Source: CAD feature listing. Evaluate the final solid. Frame: model axes, mm. A direction names the side the tool comes from. Round coordinates to 2 decimals unless told otherwise and drop trailing zeros. Loops run counter-clockwise (first coordinate to the right, second up) from the corner with the lowest first, then second, coordinate; pieces in that order, holes last. Notation, with made-up numbers: M 64.25,-4 L 112.25,-4 A17 ccw 112.25,14 Z; hole C 28,8 d1. An arc over 180 degrees is marked long. Answer as a JSON object with one key per item and string values.
from build123d import *

# Parameters (mm, degrees)
SKETCH2_R           = 63.5
BOSS_EXTRUDE1_DEPTH = 25.4
SHELL1_T            = -2
BOSS_EXTRUDE2_DEPTH = 23.4
CUT_EXTRUDE2_DEPTH  = 23.4


with BuildPart() as part:
    # Sketch2 → Boss-Extrude1 (new body)
    with BuildSketch(Plane(origin=(0, 0, 0), x_dir=(0, 1, 0), z_dir=(0, 0, 1))):
        with Locations(Location((0, 0, 0), (0, 0, 270))):
            Circle(SKETCH2_R)
    extrude(amount=BOSS_EXTRUDE1_DEPTH)

    # Shell1
    shell1_openings = [part.faces().sort_by_distance(p)[0] for p in [
        (0, 0, 25.4),
    ]]
    offset(amount=SHELL1_T, openings=shell1_openings, kind=Kind.INTERSECTION)

    # Sketch3 → Boss-Extrude2 (add)
    with BuildSketch(Plane.XY.offset(2)):
        with BuildLine():
            Line((32.449501385, 1.811038348), (34.452433007, 1.811038348))
            ThreePointArc((34.452433007, 1.811038348), (-34.49308373, 0.690778407), (34.352300121, -3.188961652))
            Line((34.352300121, -3.188961652), (32.343168113, -3.188961652))
            ThreePointArc((32.343168113, -3.188961652), (-32.492653095, 0.691010021), (32.449501385, 1.811038348))
        make_face()
    extrude(amount=BOSS_EXTRUDE2_DEPTH)

    # Sketch4 → Cut-Extrude2 (cut)
    with BuildSketch(Plane.XY.offset(25.4)):
        Polygon((34.352300121, -3.188961652), (63.419874831, -3.188961652), (70.082181446, -0.688961652), (63.474169078, 1.811038348), (34.452433007, 1.811038348), align=None)
    extrude(amount=-CUT_EXTRUDE2_DEPTH, mode=Mode.SUBTRACT)


solid = part.part
Item 1: Section A-A on z = 15.5. Return the cut outline in (x, y), then the cut area to 3 significant figures.
Answer sheet:
{"outline": "M 32.34,-3.19 A32.5 cw long 32.45,1.81 L 34.45,1.81 A34.5 ccw long 34.35,-3.19 Z; M 61.42,-3.19 A61.5 cw long 61.47,1.81 L 63.47,1.81 A63.5 ccw long 63.42,-3.19 Z", "area": "1,190 mm²"}
Item 2: Section C-C on x = 0. Return the cut outline in (y, z).
Answer sheet:
{"outline": "M -63.5,0 L 63.5,0 L 63.5,25.4 L 61.5,25.4 L 61.5,2 L 34.5,2 L 34.5,25.4 L 32.5,25.4 L 32.5,2 L -32.5,2 L -32.5,25.4 L -34.5,25.4 L -34.5,2 L -61.5,2 L -61.5,25.4 L -63.5,25.4 Z"}
Item 3: Pull-direction query (X, two-part tool) for faces 1 (the flat face through (-52, 33.2, 25.4)), 2 (the cylindrical face through (-61.41, 3.36, 13.54)), 3 (the cylindrical face through (-32.492, -0.703, 13.536)), 4 (the cylindrical face through (-13.77, -61.99, 12.52)); classes: pulls with the +X half, pulls with the -X half, needs draft (parallel to the pull), parting line crosses it, or undercut.
Answer sheet:
{"face 1": "needs draft", "face 2": "undercut", "face 3": "undercut", "face 4": "parting line crosses it"}
Item 4: Section D-D on x = -16. Return the cut outline in (y, z).
Answer sheet:
{"outline": "M -61.45,0 L 61.45,0 L 61.45,25.4 L 59.38,25.4 L 59.38,2 L 30.57,2 L 30.57,25.4 L 28.29,25.4 L 28.29,2 L -28.29,2 L -28.29,25.4 L -30.57,25.4 L -30.57,2 L -59.38,2 L -59.38,25.4 L -61.45,25.4 Z"}
Item 5: Contact query for flat-ended pins moving along their axis: pin 1 Ø8 at (y, z) = (44, 22) entering from +X; pin 2 Ø6 at (x, z) = (36.5, 4.5) entering from -Y; pin 3 Ø12 at (y, z) = (-43, 7) entering from +X; pin 4 Ø1 at (x, y) = (-20.5, -31) entering from -Z. Output: stop coordinate, or through.
Answer sheet:
{"pin 1": "stops at x = 49.32", "pin 2": "stops at y = -53.94", "pin 3": "stops at x = 51.61", "pin 4": "stops at z = 0"}
Item 6: Section B-B on y = 0. Return the cut outline in (x, z).
Answer sheet:
{"outline": "M -63.5,0 L 63.5,0 L 63.5,2 L -32.5,2 L -32.5,25.4 L -34.5,25.4 L -34.5,2 L -61.5,2 L -61.5,25.4 L -63.5,25.4 Z"}
Item 7: Line query: probe 1 along Y at (x, z) = (0, 10); probe 2 along X at (y, z) = (0, 14.75); probe 3 along X at (y, z) = (24.5, 8.5). Output: solid intervals per line, ascending. Write a range as from..to.
Answer sheet:
{"probe 1": "y = -63.5..-61.5, -34.5..-32.5, 32.5..34.5, 61.5..63.5", "probe 2": "x = -63.5..-61.5, -34.5..-32.5", "probe 3": "x = -58.58..-56.41, -24.29..-21.35, 21.35..24.29, 56.41..58.58"}
Item 8: Access query for faces 5 (the flat face through (-1, 1, 0)), 6 (the cylindrical face through (-34.43, 2.17, 13.54)). Directions: +Z, -Z, +X, -X, +Y, -Y. A direction counts if a zero-diameter tool reaches every point of the face in a straight line with its end or side. Return the directions, or none.
Answer sheet:
{"face 5": "-Z, +X, -X, +Y, -Y", "face 6": "+Z"}
